Model file for the job. Use its own axes, mm. Face numbers are marked on the shaded views. A direction names the side the tool comes from. Coordinates: 2 decimals unless noted, no trailing zeros. Order: outer loops, then holes, each group sorted by start corner. A loop starts at its lowest first (then second) coordinate and runs counter-clockwise, first axis right, second up.
from build123d import *

# Parameters (mm, degrees)
SKETCH1_W           = 104.5
SKETCH1_H           = 99.5
BOSS_EXTRUDE1_DEPTH = 8
CUT_EXTRUDE1_REACH  = 10
SKETCH2_R           = 9
SKETCH2_R_2         = 15
BOSS_EXTRUDE2_DEPTH = 99.5
CUT_EXTRUDE2_REACH  = 10
SKETCH4_W           = 27
SKETCH4_H           = 89.5
CUT_EXTRUDE3_REACH  = 10
SKETCH5_W           = 30
SKETCH5_H           = 28.99
CUT_EXTRUDE4_REACH  = 10
SKETCH6_R           = 3


with BuildPart() as part:
    # Sketch1 → Boss-Extrude1 (new body)
    with BuildSketch(Plane(origin=(0, 0, 0), x_dir=(1, 0, 0), z_dir=(0, 1, 0))):
        Rectangle(SKETCH1_W, SKETCH1_H)
    extrude(amount=BOSS_EXTRUDE1_DEPTH)

    # Sketch2 → Cut-Extrude1 (cut, up to next)
    with BuildSketch(Plane.XZ, mode=Mode.PRIVATE) as cut_extrude1_sk1:
        with Locations((-33.25, -10.15)):
            Circle(SKETCH2_R)
    cut_extrude1_tool1 = extrude(cut_extrude1_sk1.sketch, amount=-CUT_EXTRUDE1_REACH, mode=Mode.PRIVATE) & part.part
    add(cut_extrude1_tool1.solids().sort_by_distance((-33.25, 0, -10.15))[0], mode=Mode.SUBTRACT)
    # Sketch2 → Cut-Extrude1 (cut, up to next)
    with BuildSketch(Plane.XZ, mode=Mode.PRIVATE) as cut_extrude1_sk2:
        with Locations((-33.25, -35.55)):
            Circle(SKETCH2_R)
    cut_extrude1_tool2 = extrude(cut_extrude1_sk2.sketch, amount=-CUT_EXTRUDE1_REACH, mode=Mode.PRIVATE) & part.part
    add(cut_extrude1_tool2.solids().sort_by_distance((-33.25, 0, -35.55))[0], mode=Mode.SUBTRACT)
    # Sketch2 → Cut-Extrude1 (cut, up to next)
    with BuildSketch(Plane.XZ, mode=Mode.PRIVATE) as cut_extrude1_sk3:
        with Locations((34.25, 12.7)):
            Circle(SKETCH2_R)
    cut_extrude1_tool3 = extrude(cut_extrude1_sk3.sketch, amount=-CUT_EXTRUDE1_REACH, mode=Mode.PRIVATE) & part.part
    add(cut_extrude1_tool3.solids().sort_by_distance((34.25, 0, 12.7))[0], mode=Mode.SUBTRACT)
    # Sketch2 → Cut-Extrude1 (cut, up to next)
    with BuildSketch(Plane.XZ, mode=Mode.PRIVATE) as cut_extrude1_sk4:
        with Locations((34.25, -12.7)):
            Circle(SKETCH2_R)
    cut_extrude1_tool4 = extrude(cut_extrude1_sk4.sketch, amount=-CUT_EXTRUDE1_REACH, mode=Mode.PRIVATE) & part.part
    add(cut_extrude1_tool4.solids().sort_by_distance((34.25, 0, -12.7))[0], mode=Mode.SUBTRACT)
    # Sketch2 → Cut-Extrude1 (cut, up to next)
    with BuildSketch(Plane.XZ, mode=Mode.PRIVATE) as cut_extrude1_sk5:
        with Locations((-31.25, 15.76)):
            Circle(SKETCH2_R_2)
    cut_extrude1_tool5 = extrude(cut_extrude1_sk5.sketch, amount=-CUT_EXTRUDE1_REACH, mode=Mode.PRIVATE) & part.part
    add(cut_extrude1_tool5.solids().sort_by_distance((-31.25, 0, 15.76))[0], mode=Mode.SUBTRACT)

    # Sketch3 → Boss-Extrude2 (add)
    with BuildSketch(Plane(origin=(0, 0, -49.75), x_dir=(-1, 0, 0), z_dir=(0, 0, -1))):
        Polygon((6.25, 8), (10, 20), (12.5, 20), (16.25, 8), align=None)
    extrude(amount=-BOSS_EXTRUDE2_DEPTH)

    # Sketch4 → Cut-Extrude2 (cut, up to next)
    with BuildSketch(Plane(origin=(0, 8, 0), x_dir=(1, 0, 0), z_dir=(0, 1, 0)), mode=Mode.PRIVATE) as cut_extrude2_sk1:
        with Locations((7.75, 0)):
            Rectangle(SKETCH4_W, SKETCH4_H)
    cut_extrude2_tool1 = extrude(cut_extrude2_sk1.sketch, amount=-CUT_EXTRUDE2_REACH, mode=Mode.PRIVATE) & part.part
    add(cut_extrude2_tool1.solids().sort_by_distance((7.75, 8, 0))[0], mode=Mode.SUBTRACT)

    # Sketch5 → Cut-Extrude3 (cut, up to next)
    with BuildSketch(Plane(origin=(0, 8, 0), x_dir=(1, 0, 0), z_dir=(0, 1, 0)), mode=Mode.PRIVATE) as cut_extrude3_sk1:
        with Locations((-31.25, -30.255)):
            Rectangle(SKETCH5_W, SKETCH5_H)
    cut_extrude3_tool1 = extrude(cut_extrude3_sk1.sketch, amount=-CUT_EXTRUDE3_REACH, mode=Mode.PRIVATE) & part.part
    add(cut_extrude3_tool1.solids().sort_by_distance((-31.25, 8, 30.255))[0], mode=Mode.SUBTRACT)

    # Sketch6 → Cut-Extrude4 (cut, up to next)
    with BuildSketch(Plane(origin=(0, 8, 0), x_dir=(1, 0, 0), z_dir=(0, 1, 0)), mode=Mode.PRIVATE) as cut_extrude4_sk1:
        with Locations((-45.25, 42.75)):
            Circle(SKETCH6_R)
    cut_extrude4_tool1 = extrude(cut_extrude4_sk1.sketch, amount=-CUT_EXTRUDE4_REACH, mode=Mode.PRIVATE) & part.part
    add(cut_extrude4_tool1.solids().sort_by_distance((-45.25, 8, -42.75))[0], mode=Mode.SUBTRACT)
    # Sketch6 → Cut-Extrude4 (cut, up to next)
    with BuildSketch(Plane(origin=(0, 8, 0), x_dir=(1, 0, 0), z_dir=(0, 1, 0)), mode=Mode.PRIVATE) as cut_extrude4_sk2:
        with Locations((45.25, 42.75)):
            Circle(SKETCH6_R)
    cut_extrude4_tool2 = extrude(cut_extrude4_sk2.sketch, amount=-CUT_EXTRUDE4_REACH, mode=Mode.PRIVATE) & part.part
    add(cut_extrude4_tool2.solids().sort_by_distance((45.25, 8, -42.75))[0], mode=Mode.SUBTRACT)


solid = part.part
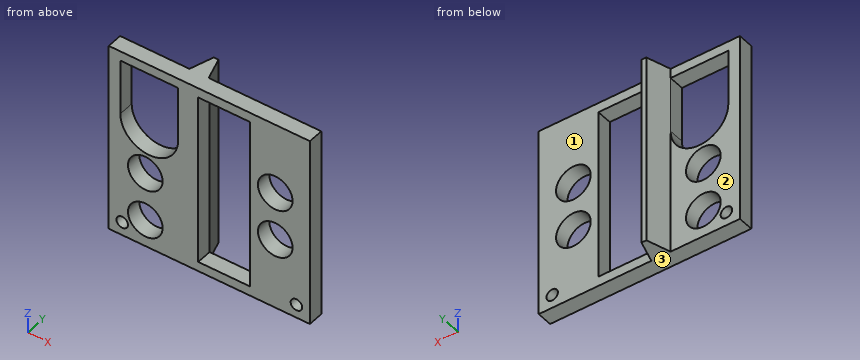
Q1. Cut at B-B, the plane z = -35.55. List the corners of the cut face in (x, y), plus the area to 3 significant figures.
Established:
outline: (-52.25, 0) - (-42.25, 0) - (-42.25, 8) - (-52.25, 8) - close; (-24.25, 0) - (-5.75, 0) - (-5.75, 8) - (-6.25, 8) - (-10, 20) - (-12.5, 20) - (-16.25, 8) - (-24.25, 8) - close; (21.25, 0) - (52.25, 0) - (52.25, 8) - (21.25, 8) - close
area: 551 mm2
Q2. Probe line 1 (Z direction, x = 34.25, y = 4.25); line 2 (X direction, y = 1.25, z = 30); line 3 (X direction, y = 2.75, z = -42.75). List the from-to ranges inside material, lowest first.
Established:
line 1: z = -49.75 to -21.7, -3.7 to 3.7, 21.7 to 49.75
line 2: x = -52.25 to -46.25, -16.25 to -5.75, 21.25 to 52.25
line 3: x = -52.25 to -48.25, -42.25 to -38.65, -27.85 to -5.75, 21.25 to 42.25, 48.25 to 52.25
Q3. Cut at C-C, the plane y = 6. Count the separate pieces of the cut face and the enclosed holes in it, plus the area to 3 significant figures.
Established:
separate pieces: 1
enclosed holes: 8
area: 5,680 mm2
Q4. Drop flat-ended pins along their axis: P1, Ø6, axis at x = 28, y = 12.5, coming from the -Z side; P2, Ø12, axis at y = 15, z = 22, coming from the +X side; P3, Ø11, axis at x = -29, z = 1, coming from the +Y side. Give the stop position or say it passes through.
Established:
P1: passes through
P2: stops at x = -6.56
P3: stops at y = 8
Q5. Cut at A-A, the plane x = 45.25. List the corners of the cut face in (y, z).
Established:
outline: (0, -49.75) - (8, -49.75) - (8, -45.75) - (0, -45.75) - close; (0, -39.75) - (8, -39.75) - (8, 49.75) - (0, 49.75) - close
Q6. Cut at D-D, the plane x = 34.25. List the corners of the cut face in (y, z).
Established:
outline: (0, -49.75) - (8, -49.75) - (8, -21.7) - (0, -21.7) - close; (0, -3.7) - (8, -3.7) - (8, 3.7) - (0, 3.7) - close; (0, 21.7) - (8, 21.7) - (8, 49.75) - (0, 49.75) - close
Q7. Which spindle directions (+Z, -Z, +X, -X, +Y, -Y) get a long thin tool onto all of the face, cutting with end or side? Do the marked faces 1, 2 and 3. Say none if no direction does.
Established:
face 1: +Z, -Z, +X, +Y
face 2: +Z, -Z, -X, +Y
face 3: -Z, +X, -X, +Y, -Y
